For this review, take the finished solid that the model builds, in its own axes (mm). Face numbers are marked on the shaded views. A direction names the side the tool comes from. Round coordinates to 2 decimals unless told otherwise and drop trailing zeros. Write each loop counter-clockwise with the first axis right and the second up, starting at its lowest first coordinate (ties: lowest second). Pieces come first, ordered by that corner, then holes. Notation, with made-up numbers: (-20, -26.5) -> (34, -26.5) arc R24 ccw to (34, -16.5) -> close; hole circle Ø9 at (86.25, -2.75). An arc over 180 degrees is marked (long way). Answer as CSV lines item,"result". Start each with the question number.
Item 1: Mouldability with a two-part tool opening along Y and no side actions: class the marked faces 1, 2, 3 and 4 as +Y half, -Y half, draft (parallel to the pull), parting line (faces both ways), or undercut.
Item 2: For pin 1 Ø4.5 at (y, z) = (42.52, 258.16) entering from +X; pin 2 Ø8 at (y, z) = (9.5, 246) entering from -X; pin 3 Ø1.6 at (x, z) = (104, 266) entering from +Y; pin 4 Ø2 at (x, y) = (99, 25.5) entering from -Z, all flat-tipped, find the tip position at first contact; note any pin that passes through.
Item 3: Machinability: for the marked faces 5 and 6, which of the approach directions +Z, -Z, +X, -X, +Y, -Y give a long, thin tool a straight path to every point of the face, cutting with its end or side? Answer none if there is none.
Item 4: Take a section at B-B on z = 228. Count the separate pieces of the cut face and the enclosed holes in it, then the cut area to 3 significant figures.
Item 5: Take a section at A-A on y = 7. Give the boundary of the cut face in (x, z), then the cut area to 3 significant figures.
Item 6: Wall thickness on probe 1 along Y at (x, z) = (97, 231); probe 2 along X at (y, z) = (22.5, 259); probe 3 along Y at (x, z) = (104.25, 238.5): over which ranges is each line inside the solid? List them lowest first. Write a range as from..to.
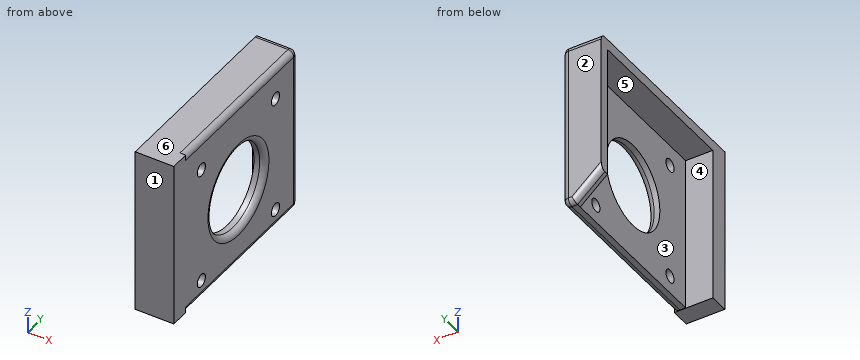
```python
from build123d import *

# Parameters (mm, degrees)
SKETCH_1_W            = 5
SKETCH_1_H            = 60
SKETCH_1_W_2          = 30
SKETCH_1_H_2          = 5
SKETCH_1_W_3          = 15
EXTRUDE_1_DEPTH       = 5
FILLET_1_R            = 5
SKETCH_2_W            = 245
SKETCH_2_H            = 125
CUT_EXTRUDE_1_DEPTH   = 5
SKETCH_3_W            = 110
SKETCH_3_H            = 2.5
SKETCH_3_W_2          = 115
CUT_EXTRUDE_2_DEPTH   = 10
SKETCH_4_W            = 5
SKETCH_4_H            = 5
CUT_EXTRUDE_3_DEPTH   = 5
SKETCH_5_W            = 50
SKETCH_5_H            = 46.65
EXTRUDE_2_DEPTH       = 47
SKETCH_6_W            = 41.4
SKETCH_6_H            = 44.05
CUT_EXTRUDE_4_DEPTH   = 47
SKETCH_7_R            = 11.25
CUT_EXTRUDE_5_DEPTH   = 317.004529962
CUT_EXTRUDE_6_DEPTH   = 46.65
SKETCH_10_R           = 1.7
CUT_EXTRUDE_7_DEPTH   = 317.004529962
SKETCH_13_R           = 25
CUT_EXTRUDE_9_DEPTH   = 20
FILLET_11_R           = 1.497
SKETCH_17_OUTSIDE_W   = 295.14
SKETCH_17_OUTSIDE_H   = 275.14
SKETCH_17_OUTSIDE_W_2 = 10.174383679
SKETCH_17_OUTSIDE_H_2 = 44.104202059
CUT_EXTRUDE_11_DEPTH  = 359.196699


with BuildPart() as part:
    # 草圖1 → 填料-伸長1 (new body)
    with BuildSketch(Plane(origin=(0, 0, 0), x_dir=(1, 0, 0), z_dir=(0, 1, 0))):
        Polygon((198.746286718, -286.464902661), (198.746286718, -256.464902661), (183.246286718, -256.464902661), (183.246286718, -266.464902661), (124.746286718, -266.464902661), (124.746286718, -262.464902661), (109.246286718, -262.464902661), (109.246286718, -266.464902661), (-21.253713282, -266.464902661), (-21.253713282, 38.535097339), (-36.253713282, 38.535097339), (-36.253713282, 43.535097339), (203.746286718, 43.535097339), (203.746286718, -286.464902661), align=None)
        with Locations((206.246286718, -256.464902661)):
            Rectangle(SKETCH_1_W, SKETCH_1_H)
        with Locations((206.246286718, 13.535097339)):
            Rectangle(SKETCH_1_W, SKETCH_1_H)
        with Locations((188.746286718, 46.035097339)):
            Rectangle(SKETCH_1_W_2, SKETCH_1_H_2)
        with Locations((-21.253713282, 46.035097339)):
            Rectangle(SKETCH_1_W_2, SKETCH_1_H_2)
        with Locations((91.246286718, 46.035097339)):
            Rectangle(SKETCH_1_W_3, SKETCH_1_H_2)
        with Locations((76.246286718, 46.035097339)):
            Rectangle(SKETCH_1_W_3, SKETCH_1_H_2)
        with Locations((206.246286718, -166.464902661)):
            Rectangle(SKETCH_1_W, SKETCH_1_H)
        with Locations((206.246286718, -76.464902661)):
            Rectangle(SKETCH_1_W, SKETCH_1_H)
    extrude(amount=EXTRUDE_1_DEPTH)

    # 圓角1
    fillet_1_edges = [part.edges().sort_by_distance(p)[0] for p in [
        (208.746286718, 5, -13.535097339),
        (208.746286718, 5, 76.464902661),
        (208.746286718, 5, 166.464902661),
        (208.746286718, 5, 256.464902661),
    ]]
    fillet(fillet_1_edges, radius=FILLET_1_R - 0.0001)  # a hair under: the kernel refuses the full size

    # 草圖2 → 除料-伸長1 (cut)
    with BuildSketch(Plane(origin=(0, 5, 0), x_dir=(1, 0, 0), z_dir=(0, 1, 0))):
        with Locations((86.246286718, -13.964902661)):
            Rectangle(SKETCH_2_W, SKETCH_2_H)
    extrude(amount=-CUT_EXTRUDE_1_DEPTH, mode=Mode.SUBTRACT)

    # 草圖3 → 除料-伸長2 (cut)
    with BuildSketch(Plane(origin=(0, 0, 76.464902661), x_dir=(-1, 0, 0), z_dir=(0, 0, -1))):
        with Locations((-33.746286718, 1.25)):
            Rectangle(SKETCH_3_W, SKETCH_3_H)
        with Locations((-151.246286718, 3.75)):
            Rectangle(SKETCH_3_W_2, SKETCH_3_H)
    extrude(amount=-CUT_EXTRUDE_2_DEPTH, mode=Mode.SUBTRACT)

    # 草圖4 → 除料-伸長3 (cut)
    with BuildSketch(Plane(origin=(0, 0, 76.464902661), x_dir=(-1, 0, 0), z_dir=(0, 0, -1))):
        with Locations((-91.246286718, 2.5)):
            Rectangle(SKETCH_4_W, SKETCH_4_H)
    extrude(amount=-CUT_EXTRUDE_3_DEPTH, mode=Mode.SUBTRACT)

    # 草圖5 → 填料-伸長2 (add)
    with BuildSketch(Plane.XY.offset(266.464902661)):
        with Locations((79.746286718, 28.325)):
            Rectangle(SKETCH_5_W, SKETCH_5_H)
    extrude(amount=-EXTRUDE_2_DEPTH)

    # 草圖6 → 除料-伸長4 (cut)
    with BuildSketch(Plane.ZY.offset(-54.746286718)):
        with Locations((242.964902661, 27.025)):
            Rectangle(SKETCH_6_W, SKETCH_6_H)
    extrude(amount=-CUT_EXTRUDE_4_DEPTH, mode=Mode.SUBTRACT)

    # 草圖7 → 除料-伸長5 (cut, through all)
    with BuildSketch(Plane.ZY.offset(-101.746286718)):
        with Locations((242.664902661, 27.025)):
            Circle(SKETCH_7_R)
    extrude(amount=-CUT_EXTRUDE_5_DEPTH, mode=Mode.SUBTRACT)

    # 草圖8 → 除料-伸長6 (cut)
    with BuildSketch(Plane(origin=(0, 51.65, 0), x_dir=(1, 0, 0), z_dir=(0, 1, 0))):
        Polygon((54.746286718, -263.664902661), (101.746286718, -222.464902661), (104.746286718, -222.464902661), (104.746286718, -219.464902661), (54.746286718, -219.464902661), align=None)
    extrude(amount=-CUT_EXTRUDE_6_DEPTH, mode=Mode.SUBTRACT)

    # 草圖10 → 除料-伸長7 (cut, through all)
    with BuildSketch(Plane.ZY.offset(-101.746286718)):
        with Locations((227.164902661, 42.525)):
            Circle(SKETCH_10_R)
        with Locations((258.164902661, 42.525)):
            Circle(SKETCH_10_R)
        with Locations((258.164902661, 11.525)):
            Circle(SKETCH_10_R)
        with Locations((227.164902661, 11.525)):
            Circle(SKETCH_10_R)
    extrude(amount=-CUT_EXTRUDE_7_DEPTH, mode=Mode.SUBTRACT)

    # 草圖13 → 除料-伸長9 (cut)
    with BuildSketch(Plane(origin=(104.746286718, 0, 0), x_dir=(0, 0, -1), z_dir=(1, 0, 0))):
        with Locations((-242.664902661, 27.025)):
            Circle(SKETCH_13_R)
    extrude(amount=CUT_EXTRUDE_9_DEPTH, mode=Mode.SUBTRACT)

    # 圓角11
    fillet_11_edges = [part.edges().sort_by_distance(p)[0] for p in [
        (54.746286718, 28.325, 266.464902661),
        (79.746286718, 51.65, 266.464902661),
        (104.746286718, 28.325, 266.464902661),
        (104.746286718, 27.025, 231.414902661),
        (54.746286718, 51.65, 265.064902661),
        (104.746286718, 51.65, 244.464902661),
        (104.746286718, 28.325, 222.464902661),
        (78.246286718, 51.65, 243.064902661),
        (103.246286718, 51.65, 222.464902661),
    ]]
    fillet(fillet_11_edges, radius=FILLET_11_R)

    # 草圖17 outside → 除料-伸長11 (cut, through all)
    with BuildSketch(Plane(origin=(0, 51.65, 0), x_dir=(1, 0, 0), z_dir=(0, 1, 0))):
        with Locations((93.746, -181.465)):
            Rectangle(SKETCH_17_OUTSIDE_W, SKETCH_17_OUTSIDE_H)
        with Locations((99.659094879, -244.412801632)):
            Rectangle(SKETCH_17_OUTSIDE_W_2, SKETCH_17_OUTSIDE_H_2, mode=Mode.SUBTRACT)
    extrude(amount=-CUT_EXTRUDE_11_DEPTH, mode=Mode.SUBTRACT)


solid = part.part
```
Output values:
1,face 1,"-Y half"
1,face 2,"+Y half"
1,face 3,"undercut"
1,face 4,"undercut"
2,pin 1,"stops at x = 104.75"
2,pin 2,"stops at x = 101.75"
2,pin 3,"stops at y = 51.57"
2,pin 4,"stops at z = 263.66"
3,face 5,"-Z, -X"
3,face 6,"+Z, +X, -X, +Y, -Y"
4,separate pieces,"3"
4,enclosed holes,"0"
4,area,"188 mm^2"
5,outline,"(94.57, 263.66) -> (101.75, 263.66) -> (101.75, 222.46) -> (103.25, 222.46) arc R1.5 ccw to (104.75, 223.96) -> (104.75, 264.97) arc R1.5 ccw to (103.25, 266.46) -> (94.57, 266.46) -> close"
5,area,"151 mm^2"
6,probe 1,"y = 0..5, 49.05..51.65"
6,probe 2,"x = 101.75..104.75"
6,probe 3,"y = 0..16.16, 37.89..51.27"
